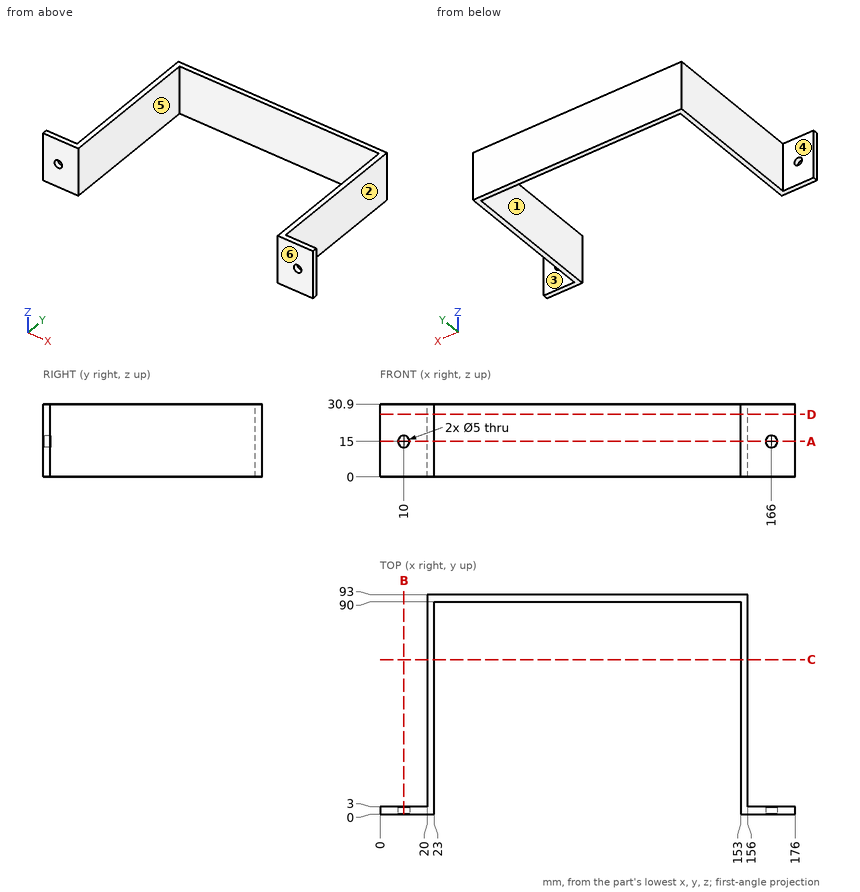
Can you work these out from the drawing? Everything is in mm from the part's minimum corner. A direction names the side the tool comes from. Give positions to 0.01 mm unless a question says otherwise; leave off trailing zeros. Loops run counter-clockwise (first coordinate to the right, second up) from the corner with the lowest first, then second, coordinate; pieces in that order, holes last. Notation, with made-up numbers: (6, 50.25) - (36, 50.25) arc R27 cw to (36, 80.25) - close; hole circle Ø10 at (-31.75, 54). An arc over 180 degrees is marked (long way). Use one line per item in the form item = value.
1. I want a section at B-B (x = 10). Please give me the cut outline in (y, z), and give its area (3 significant figures).
Response values:
outline = (0, 0) - (3, 0) - (3, 12.5) - (0, 12.5) - close; (0, 17.5) - (3, 17.5) - (3, 30.9) - (0, 30.9) - close
area = 77.7 mm²
2. I want a section at C-C (y = 65.5). Please give me the cut outline in (x, z), and give its area (3 significant figures).
Response values:
outline = (20, 0) - (23, 0) - (23, 30.9) - (20, 30.9) - close; (153, 0) - (156, 0) - (156, 30.9) - (153, 30.9) - close
area = 185 mm²
3. I'm going to push flat-ended pins straight in: pin 1 Ø9.5 at (y, z) = (51, 16) entering from -X; pin 2 Ø2 at (y, z) = (24.5, 20.5) entering from +X; pin 3 Ø4 at (x, z) = (129, 7.5) entering from -Y. Where does each tip first touch, or does it pass through?
Response values:
pin_1 = 20
pin_2 = 156
pin_3 = 90
4. Thinking about a two-plate mould opening in X: for the marked faces 1, 2 and 3, which applies, released by +X, released by -X, zero draft, split by the parting line, or undercut?
Response values:
face_1 = undercut
face_2 = released by +X
face_3 = zero draft
5. I need wall thicknesses on probe 1 along X at (y, z) = (2, 15); probe 2 along X at (y, z) = (61, 12.5); probe 3 along Z at (x, y) = (166, 1.35). Which ranges of each line are inside material? Lowest first, please.
Response values:
probe_1 = 0 to 7.5, 12.5 to 23, 153 to 163.5, 168.5 to 176
probe_2 = 20 to 23, 153 to 156
probe_3 = 0 to 12.5, 17.5 to 30.9
6. I want a section at D-D (z = 26.5). Please give me the cut outline in (x, y).
Response values:
outline = (0, 0) - (23, 0) - (23, 90) - (153, 90) - (153, 0) - (176, 0) - (176, 3) - (156, 3) - (156, 93) - (20, 93) - (20, 3) - (0, 3) - close
7. I want a section at A-A (z = 15). Please give me the cut outline in (x, y), and give its area (3 significant figures).
Response values:
outline = (0, 0) - (7.5, 0) - (7.5, 3) - (0, 3) - close; (12.5, 0) - (23, 0) - (23, 90) - (153, 90) - (153, 0) - (163.5, 0) - (163.5, 3) - (156, 3) - (156, 93) - (20, 93) - (20, 3) - (12.5, 3) - close; (168.5, 0) - (176, 0) - (176, 3) - (168.5, 3) - close
area = 1,040 mm²
8. On a 3-axis mill with a long thin cutter (end or side, diameter ignored), from which of +Z, -Z, +X, -X, +Y, -Y can I reach the whole of each face in a straight line? I mean the marked faces 4, 5 and 6. Say none if no direction works.
Response values:
face_4 = +Z, -Z, -X, +Y
face_5 = +Z, -Z, -Y
face_6 = +Z, -Z, +X, -X, -Y
